Autodesk Inventor part; units mm, degrees
ref_plane "YZ Plane" through (0, 0, 0) normal (1, 0, 0) x (0, 1, 0)
ref_plane "XZ Plane" through (0, 0, 0) normal (0, 1, 0) x (-1, 0, 0)
ref_plane "XY Plane" through (0, 0, 0) normal (0, 0, 1) x (1, 0, 0)
sketch "Sketch1" plane through (0, 0, 0) normal (0, 0, 1) x (1, 0, 0)
  line L0 (-3.9007, 3.9007) -> (3.9007, 3.9007)
  line L1 (3.9007, 3.9007) -> (3.9007, -3.9007)
  line L2 (3.9007, -3.9007) -> (-3.9007, -3.9007)
  line L3 (-3.9007, -3.9007) -> (-3.9007, 3.9007)
  line L4 (0, 3.9007) -> (0, -3.9007) construction
  line L5 (-3.9007, 0) -> (3.9007, 0) construction
  circle A0 centre (0, 0) radius 2.1
  line L6 (0, 0) -> (-16.1173, 16.1173) construction
  line L7 (0, 0) -> (22.7933, 0) construction
  line L8 (-2.84, 3.9007) -> (-5.4993, 6.56)
  line L9 (-5.4993, 6.56) -> (-5.4993, 8.2)
  line L10 (-5.4993, 8.2) -> (-2.84, 8.2)
  line L11 (-2.84, 8.2) -> (-4.64, 10)
  line L12 (-4.64, 10) -> (-10, 10)
  line L13 (-10, 10) -> (-10, 4.64)
  line L14 (-10, 4.64) -> (-8.2, 2.84)
  line L15 (-8.2, 2.84) -> (-8.2, 5.4993)
  line L16 (-8.2, 5.4993) -> (-6.56, 5.4993)
  line L17 (-6.56, 5.4993) -> (-3.9007, 2.84)
  line L18 (-3.9007, 2.84) -> (-11.3102, 2.84) construction
  line L19 (-2.84, 3.9007) -> (-3.9007, 3.9007)
  line L20 (-3.9007, 2.84) -> (-3.9007, 3.9007)
  line L21 (-3.9007, -2.84) -> (-6.56, -5.4993)
  line L22 (-6.56, -5.4993) -> (-8.2, -5.4993)
  line L23 (-8.2, -5.4993) -> (-8.2, -2.84)
  line L24 (-8.2, -2.84) -> (-10, -4.64)
  line L25 (-10, -4.64) -> (-10, -10)
  line L26 (-10, -10) -> (-4.64, -10)
  line L27 (-4.64, -10) -> (-2.84, -8.2)
  line L28 (-2.84, -8.2) -> (-5.4993, -8.2)
  line L29 (-5.4993, -8.2) -> (-5.4993, -6.56)
  line L30 (-5.4993, -6.56) -> (-2.84, -3.9007)
  line L31 (-3.9007, -2.84) -> (-3.9007, -3.9007)
  line L32 (-2.84, -3.9007) -> (-3.9007, -3.9007)
  line L33 (2.84, -3.9007) -> (5.4993, -6.56)
  line L34 (5.4993, -6.56) -> (5.4993, -8.2)
  line L35 (5.4993, -8.2) -> (2.84, -8.2)
  line L36 (2.84, -8.2) -> (4.64, -10)
  line L37 (4.64, -10) -> (10, -10)
  line L38 (10, -10) -> (10, -4.64)
  line L39 (10, -4.64) -> (8.2, -2.84)
  line L40 (8.2, -2.84) -> (8.2, -5.4993)
  line L41 (8.2, -5.4993) -> (6.56, -5.4993)
  line L42 (6.56, -5.4993) -> (3.9007, -2.84)
  line L43 (2.84, -3.9007) -> (3.9007, -3.9007)
  line L44 (3.9007, -2.84) -> (3.9007, -3.9007)
  line L45 (3.9007, 2.84) -> (6.56, 5.4993)
  line L46 (6.56, 5.4993) -> (8.2, 5.4993)
  line L47 (8.2, 5.4993) -> (8.2, 2.84)
  line L48 (8.2, 2.84) -> (10, 4.64)
  line L49 (10, 4.64) -> (10, 10)
  line L50 (10, 10) -> (4.64, 10)
  line L51 (4.64, 10) -> (2.84, 8.2)
  line L52 (2.84, 8.2) -> (5.4993, 8.2)
  line L53 (5.4993, 8.2) -> (5.4993, 6.56)
  line L54 (5.4993, 6.56) -> (2.84, 3.9007)
  line L55 (3.9007, 2.84) -> (3.9007, 3.9007)
  line L56 (2.84, 3.9007) -> (3.9007, 3.9007)
  dimension "d7" = 4.2
  dimension "d8" = 135
  dimension "d9" = 1.5
  dimension "d10" = 1.64
  dimension "d11" = 1.8
  dimension "d12" = 2.84
  dimension "d13" = 10
  dimension "d16" = 360
extrude "Extrusion1" add sketch "Sketch1" along normal blind 500
pattern_linear "Rectangular Pattern1" count 2 spacing 20 along (0, -1, 0) of "Extrusion1"
sketch "Sketch2" plane through (0, 0, 500) normal (0, 0, 1) x (1, 0, 0)
  line L0 (8.2, -2.84) -> (8.2, -5.4993)
  line L1 (8.2, -5.4993) -> (6.56, -5.4993)
  line L2 (-6.56, -5.4993) -> (-8.2, -5.4993)
  line L3 (-8.2, -5.4993) -> (-8.2, -2.84)
  line L4 (-8.2, -14.5007) -> (-6.56, -14.5007)
  line L5 (6.56, -14.5007) -> (8.2, -14.5007)
  line L6 (5.4993, -11.8) -> (5.4993, -13.44)
  line L7 (5.4993, -13.44) -> (2.84, -16.0993)
  line L8 (-2.84, -16.0993) -> (-5.4993, -13.44)
  line L9 (-5.4993, -8.2) -> (-5.4993, -6.56)
  line L10 (-5.4993, -6.56) -> (-2.84, -3.9007)
  line L11 (2.84, -3.9007) -> (5.4993, -6.56)
  line L12 (2.84, -8.2) -> (4.64, -10)
  line L13 (-8.2, -6.9993) -> (-5.9387, -6.9993)
  line L14 (-5.9387, -6.9993) -> (-4.1231, -5.1837)
  line L15 (-4.1231, -5.1837) -> (4.1231, -5.1837)
  line L16 (4.1231, -5.1837) -> (5.9387, -6.9993)
  line L17 (5.9387, -6.9993) -> (8.2, -6.9993)
  line L18 (8.2, -6.9993) -> (8.2, -13.0007)
  line L19 (8.2, -13.0007) -> (5.9387, -13.0007)
  line L20 (5.9387, -13.0007) -> (4.2461, -14.6932)
  line L21 (4.2461, -14.6932) -> (-4.2461, -14.6932)
  line L22 (-4.2461, -14.6932) -> (-5.9387, -13.0007)
  line L23 (-5.9387, -13.0007) -> (-8.2, -13.0007)
  line L24 (-8.2, -13.0007) -> (-8.2, -6.9993)
  dimension "d23" = 1.5
  dimension "d24" = 1.5
  dimension "d25" = 1.5
  dimension "d26" = 1.5
extrude "Extrusion2" cut sketch "Sketch2" against normal up to next
equation "\"d24\" = d23"
equation "\"d25\" = d23"
equation "\"d26\" = d23"
properties part number "20x40x500mm"
The listing builds one solid part. Answer for the finished solid, in the listing's coordinates (mm). Round coordinates to 2 decimals unless told otherwise and drop trailing zeros. Use a Markdown table: item, result. Add a question column.
1. Consider line 1 (Y direction, x = 0, z = 319); line 2 (Y direction, x = 6.5, z = 38.5); line 3 (X direction, y = 7, z = 130). Determine where each line is inside the solid, lowest interval first.
2. The part is cut by section A-A (z = 251). Give the number of separate pieces and of enclosed holes in the cut face, and give its area (3 significant figures).
3. Flat-ended cylindrical pins translate along their axes: P1, Ø2, axis at y = -23, z = 103.5, coming from the +X side; P2, Ø0.8, axis at y = 4.5, z = 339, coming from the +X side; P3, Ø1.5, axis at y = -2.5, z = 242, coming from the +X side; P4, Ø1.7, axis at y = -18.5, z = 256.5, coming from the +X side. Find the tip coordinate at first contact, or state that the pin passes through.
Reported:
| question | item | result |
|---|---|---|
| 1 | line 1 | -23.9 to -22.1, -17.9 to -16.1, -3.9 to -2.1, 2.1 to 3.9 |
| 1 | line 2 | -30 to -25.44, -14.56 to -13, -7 to -5.44, 5.44 to 10 |
| 1 | line 3 | -10 to -5.5, 5.5 to 10 |
| 2 | separate pieces | 1 |
| 2 | enclosed holes | 3 |
| 2 | area | 297 mm^2 |
| 3 | P1 | x = 9.36 |
| 3 | P2 | x = 10 |
| 3 | P3 | x = 8.61 |
| 3 | P4 | x = 3.9 |
